Autodesk Inventor part; units mm, degrees
ref_plane "YZ Plane" through (0, 0, 0) normal (1, 0, 0) x (0, 1, 0)
ref_plane "XZ Plane" through (0, 0, 0) normal (0, 1, 0) x (-1, 0, 0)
ref_plane "XY Plane" through (0, 0, 0) normal (0, 0, 1) x (1, 0, 0)
sketch "Sketch_1" plane through (0, 0, 0) normal (1, 0, 0) x (0, 1, 0)
  line L0 (0, 80) -> (0, 0)
  line L1 (0, 0) -> (80, 0)
  arc A0 (80, 0) -> (74, 6) centre (74, 0) ccw
  line L2 (74, 6) -> (14, 6)
  arc A1 (6, 14) -> (14, 6) centre (14, 14) ccw
  line L3 (6, 14) -> (6, 74)
  arc A2 (6, 74) -> (0, 80) centre (0, 74) ccw
extrude "Extrusion1" add sketch "Sketch_1" along normal mid plane 76
sketch "Sketch2" plane through (38, 80, 0) normal (0, 0, -1) x (-1, 0, 0)
  point P0 (18, -20)
hole "Hole1" at (20, 60, 0) direction (0, 0, 1) diameter 8.3 depth 6.6
sketch "Sketch3" plane through (38, 80, 0) normal (0, 0, -1) x (-1, 0, 0)
  point P0 (58, -60)
hole "Hole2" at (-20, 20, 0) direction (0, 0, 1) diameter 8.3 depth 6.6
sketch "Sketch4" plane through (38, 80, 0) normal (0, 0, -1) x (-1, 0, 0)
  point P0 (58, -20)
hole "Hole3" at (-20, 60, 0) direction (0, 0, 1) diameter 8.3 depth 6.6
sketch "Sketch5" plane through (-38, 0, 0) normal (0, -1, 0) x (1, 0, 0)
  point P0 (58, 20)
hole "Hole4" at (20, 0, 20) direction (0, 1, 0) diameter 8.3 depth 6.6
sketch "Sketch6" plane through (-38, 0, 0) normal (0, -1, 0) x (1, 0, 0)
  point P0 (58, 60)
hole "Hole5" at (20, 0, 60) direction (0, 1, 0) diameter 8.3 depth 6.6
sketch "Sketch7" plane through (-38, 0, 0) normal (0, -1, 0) x (1, 0, 0)
  point P0 (18, 20)
hole "Hole6" at (-20, 0, 20) direction (0, 1, 0) diameter 8.3 depth 6.6
sketch "Sketch8" plane through (-38, 0, 0) normal (0, -1, 0) x (1, 0, 0)
  point P0 (18, 60)
hole "Hole7" at (-20, 0, 60) direction (0, 1, 0) diameter 8.3 depth 6.6
sketch "Sketch9" plane through (38, 80, 0) normal (0, 0, -1) x (-1, 0, 0)
  point P0 (18, -60)
hole "Hole8" at (20, 20, 0) direction (0, 0, 1) diameter 8.3 depth 6.6
properties part number "40-4304 Aluminum"
Could you check a few things on this model? Use its own coordinates, in mm. A direction names the side the tool comes from. Give positions to 0.01 mm unless a question says otherwise; leave off trailing zeros. Loops run counter-clockwise (first coordinate to the right, second up) from the corner with the lowest first, then second, coordinate; pieces in that order, holes last. Notation, with made-up numbers: (83.25, -15.75) - (125.25, -15.75) arc R21 cw to (125.25, 7.25) - close; hole circle Ø9 at (84.25, -1.5). An arc over 180 degrees is marked (long way). Answer in a Markdown table with one row per item. Add a question column.
Q1. If we section it at D-D (x = 6): List the corners of the cut face in (y, z) for me, plus the area to 3 significant figures.
Q2. If we section it at C-C (x = 20): List the corners of the cut face in (y, z) for me, plus the area to 3 significant figures.
Q3. If we section it at A-A (z = 60): List the corners of the cut face in (x, y) for me, plus the area to 3 significant figures.
Q4. Please list where these lines run through material, in increasing order: L1, parallel to X at y = 2.05, z = 60; L2, parallel to Z at x = -4, y = 20; L3, parallel to Y at x = 20, z = 3. Write a range as from..to.
Q5. We'd pull the mould along X, two halves only. Please class faces 3 (the face through (22.53, 16.71, 3.04)), 4 (the face through (-1, 6, 44)), 5 (the face through (38, 4, 22)), 6 (the face through (-38, 4, 22)): +X half, -X half, draft (parallel to the pull), parting line (faces both ways), or undercut.
Q6. Which directions (+Z, -Z, +X, -X, +Y, -Y) give clear straight access to the entire face, cutting with the end or side of a thin tool? Please do faces 1 (the face through (-1, 44, 6)), 2 (the face through (22.53, 56.71, 3.04)).
Q7. For pin 1 (1.5 mm diameter, centred on x = 24, z = 35, fed in from -Y); pin 2 (1 mm diameter, centred on x = 1, y = 52, fed in from +Z); pin 3 (11 mm diameter, centred on x = -20, z = 60, fed in from +Y), each with a flat end and sliding along its axis, tell me the tip position at first contact or that it passes through.
The answers:
| question | item | result |
|---|---|---|
| 1 | outline | (0, 0) - (80, 0) arc R6 ccw to (74, 6) - (14, 6) arc R8 cw to (6, 14) - (6, 74) arc R6 ccw to (0, 80) - close |
| 1 | area | 922 mm^2 |
| 2 | outline | (0, 0) - (15.85, 0) - (15.85, 6) - (14, 6) arc R8 cw to (6, 14) - (6, 15.85) - (0, 15.85) - close; (0, 24.15) - (6, 24.15) - (6, 55.85) - (0, 55.85) - close; (0, 64.15) - (6, 64.15) - (6, 74) arc R6 ccw to (0, 80) - close; (24.15, 0) - (55.85, 0) - (55.85, 6) - (24.15, 6) - close; (64.15, 0) - (80, 0) arc R6 ccw to (74, 6) - (64.15, 6) - close |
| 2 | area | 723 mm^2 |
| 3 | outline | (-38, 0) - (-24.15, 0) - (-24.15, 6) - (-38, 6) - close; (-15.85, 0) - (15.85, 0) - (15.85, 6) - (-15.85, 6) - close; (24.15, 0) - (38, 0) - (38, 6) - (24.15, 6) - close |
| 3 | area | 356 mm^2 |
| 4 | L1 | x = -38..-24.15, -15.85..15.85, 24.15..38 |
| 4 | L2 | z = 0..6 |
| 4 | L3 | y = 0..15.85, 24.15..55.85, 64.15..79.2 |
| 5 | face 3 | undercut |
| 5 | face 4 | draft |
| 5 | face 5 | +X half |
| 5 | face 6 | -X half |
| 6 | face 1 | +Z, +X, -X, +Y |
| 6 | face 2 | +Z, -Z |
| 7 | pin 1 | stops at y = 0 |
| 7 | pin 2 | stops at z = 6 |
| 7 | pin 3 | stops at y = 6 |
